from build123d import *

# Parameters (mm, degrees)
SKETCH1_W           = 50
SKETCH1_H           = 60
BOSS_EXTRUDE1_DEPTH = 10
CUT_EXTRUDE1_DEPTH  = 4
SKETCH3_W           = 23
SKETCH3_H           = 10.5
SKETCH3_W_2         = 21
SKETCH3_H_2         = 8.5
CUT_EXTRUDE2_DEPTH  = 10
SKETCH4_W           = 9
SKETCH4_H           = 43.8
CUT_EXTRUDE3_DEPTH  = 2.5
SKETCH5_W           = 35
SKETCH5_H           = 19
CUT_EXTRUDE4_DEPTH  = 1.5
SKETCH6_W           = 12.3
SKETCH6_H           = 6.8
CUT_EXTRUDE5_DEPTH  = 1.5
FILLET1_R           = 2


with BuildPart() as part:
    # Sketch1 → Boss-Extrude1 (new body)
    with BuildSketch(Plane(origin=(0, 0, 0), x_dir=(1, 0, 0), z_dir=(0, 1, 0))):
        Rectangle(SKETCH1_W, SKETCH1_H)
    extrude(amount=BOSS_EXTRUDE1_DEPTH)

    # Sketch2 → Cut-Extrude1 (cut)
    with BuildSketch(Plane(origin=(0, 10, 0), x_dir=(1, 0, 0), z_dir=(0, 1, 0))):
        Polygon((-22.75, 27.975), (22.75, 27.975), (22.75, -17.025), (13.25, -17.025), (13.25, -27.22), (-13.25, -27.22), (-13.25, -17.025), (-22.75, -17.025), align=None)
    extrude(amount=-CUT_EXTRUDE1_DEPTH, mode=Mode.SUBTRACT)

    # Sketch3 → Cut-Extrude2 (cut)
    with BuildSketch(Plane.XZ):
        with Locations((0, -22.5)):
            Rectangle(SKETCH3_W, SKETCH3_H)
        with Locations((0, 21.72)):
            Rectangle(SKETCH3_W_2, SKETCH3_H_2)
    extrude(amount=-CUT_EXTRUDE2_DEPTH, mode=Mode.SUBTRACT)

    # Sketch4 → Cut-Extrude3 (cut)
    with BuildSketch(Plane(origin=(0, 6, 0), x_dir=(1, 0, 0), z_dir=(0, 1, 0))):
        with Locations((-17.793551609, 5.475)):
            Rectangle(SKETCH4_W, SKETCH4_H)
        with Locations((17.838749051, 5.475)):
            Rectangle(SKETCH4_W, SKETCH4_H)
    extrude(amount=-CUT_EXTRUDE3_DEPTH, mode=Mode.SUBTRACT)

    # Sketch5 → Cut-Extrude4 (cut)
    with BuildSketch(Plane.XZ):
        with Locations((0, -6)):
            Rectangle(SKETCH5_W, SKETCH5_H)
    extrude(amount=-CUT_EXTRUDE4_DEPTH, mode=Mode.SUBTRACT)

    # Sketch6 → Cut-Extrude5 (cut)
    with BuildSketch(Plane.XZ):
        with Locations((0, 10)):
            Rectangle(SKETCH6_W, SKETCH6_H)
    extrude(amount=-CUT_EXTRUDE5_DEPTH, mode=Mode.SUBTRACT)

    # Fillet1
    fillet1_edges = [part.edges().sort_by_distance(p)[0] for p in [
        (25, 5, 30),
        (-25, 5, 30),
        (-25, 5, -30),
        (25, 5, -30),
    ]]
    fillet(fillet1_edges, radius=FILLET1_R)


solid = part.part
Work out the finished part from the listing and answer in its coordinate system (mm). A direction names the side the tool comes from. Round coordinates to 2 decimals unless told otherwise and drop trailing zeros. Write each loop counter-clockwise with the first axis right and the second up, starting at its lowest first coordinate (ties: lowest second). Pieces come first, ordered by that corner, then holes.
1) A cutting plane is placed at D-D (z = 10). Give the vertices of the cut face in (x, y).
2) A cutting plane is placed at C-C (y = 7.25). Give the vertices of the cut face in (x, z) (3 decimals).
3) Given pin 1 Ø4.5 at (x, z) = (-15.5, -12) entering from +Y; pin 2 Ø3 at (x, z) = (8.5, -3.5) entering from -Y, each flat-ended and moving along its own axis, determine where each tip first touches the part or whether it passes through.
4) The mould has two halves that part along X. Classify faces 1 (the flat face through (-15, 10, 18)), 2 (the cylindrical face through (-24.43, 5.07, 29.4)), 3 (the flat face through (18, 8, 17.025)), 4 (the flat face through (0, 3, 17.47)): pulls with the +X half, pulls with the -X half, needs draft (parallel to the pull), parting line crosses it, or undercut.
5) A cutting plane is placed at A-A (z = 21). Give the vertices of the cut face in (x, y).
6) A cutting plane is placed at B-B (x = 4). Give the vertices of the cut face in (y, z) (3 decimals), plus the area to 3 significant figures.
7) Straight lines are drawn through the part: line 1 (Z direction, x = 10, y = 5.5); line 2 (X direction, y = 5.5, z = -21); line 3 (X direction, y = 4.5, z = 21). For each, find the intervals that lie inside material, in ascending order.
8) A tool of negligible diameter and unlimited length cuts with its end or side. For faces 5 (the flat face through (0, 3, 25.97)), 6 (the flat face through (0, 1, 13.4)), 7 (the flat face through (25, 5, 0)), 8 (the flat face through (-18, 3.5, -6)), from which of +Z, -Z, +X, -X, +Y, -Y can it reach the whole face along a straight path? Write none if from no direction.
Completed:
1. outline: (-25, 0) - (-6.15, 0) - (-6.15, 1.5) - (6.15, 1.5) - (6.15, 0) - (25, 0) - (25, 10) - (22.75, 10) - (22.75, 6) - (22.34, 6) - (22.34, 3.5) - (13.34, 3.5) - (13.34, 6) - (-13.29, 6) - (-13.29, 3.5) - (-22.29, 3.5) - (-22.29, 6) - (-22.75, 6) - (-22.75, 10) - (-25, 10) - close
2. outline: (-25, -28) arc R2 ccw to (-23, -30) - (23, -30) arc R2 ccw to (25, -28) - (25, 28) arc R2 ccw to (23, 30) - (-23, 30) arc R2 ccw to (-25, 28) - close; hole (-22.75, -27.975) - (22.75, -27.975) - (22.75, 17.025) - (13.25, 17.025) - (13.25, 27.22) - (-13.25, 27.22) - (-13.25, 17.025) - (-22.75, 17.025) - close
3. pin 1: stops at y = 6
3. pin 2: stops at y = 1.5
4. face 1: needs draft
4. face 2: pulls with the -X half
4. face 3: undercut
4. face 4: undercut
5. outline: (-25, 0) - (-10.5, 0) - (-10.5, 6) - (-13.25, 6) - (-13.25, 10) - (-25, 10) - close; (10.5, 0) - (25, 0) - (25, 10) - (13.25, 10) - (13.25, 6) - (10.5, 6) - close
6. outline: (0, -30) - (10, -30) - (10, -27.975) - (6, -27.975) - (6, -27.75) - (0, -27.75) - close; (0, -17.25) - (6, -17.25) - (6, 17.47) - (0, 17.47) - (0, 13.4) - (1.5, 13.4) - (1.5, 6.6) - (0, 6.6) - (0, 3.5) - (1.5, 3.5) - (1.5, -15.5) - (0, -15.5) - close; (0, 25.97) - (6, 25.97) - (6, 27.22) - (10, 27.22) - (10, 30) - (0, 30) - close
6. area: 227 mm2
7. line 1: z = -30 to -27.75, -17.25 to 17.47, 25.97 to 30
7. line 2: x = -25 to -22.29, -13.29 to -11.5, 11.5 to 13.34, 22.34 to 25
7. line 3: x = -25 to -10.5, 10.5 to 25
8. face 5: +Y, -Y
8. face 6: -Y
8. face 7: +Z, -Z, +X, +Y, -Y
8. face 8: +Y
